Work out the finished part from the listing and answer in its coordinate system (mm). A direction names the side the tool comes from. Coordinates: 2 decimals unless noted, no trailing zeros. Loops run counter-clockwise (first coordinate to the right, second up) from the corner with the lowest first, then second, coordinate; pieces in that order, holes last. Notation, with made-up numbers: M 79.25,40 L 110.25,40 A14 ccw 110.25,51 Z; hole C 5.5,38 d9. An arc over 180 degrees is marked long. Write each question's results on one line, items separated by ' | '.
```python
from build123d import *

# Parameters (mm, degrees)
SZKIC1_W                                             = 119.8
SZKIC1_H                                             = 10
DODANIE_WYCI_GNI_CIE2_DEPTH                          = 30
SZKIC21_W                                            = 119.8
SZKIC21_H                                            = 10
DODANIE_WYCI_GNI_CIE3_DEPTH                          = 9.8
POG_BIENIE_WALCOWE_POD_M2_WKR_T_DO_CZ_CI_D           = 2.4
POG_BIENIE_WALCOWE_POD_M2_WKR_T_DO_CZ_CI_CBORE_D     = 5
POG_BIENIE_WALCOWE_POD_M2_WKR_T_DO_CZ_CI_CBORE_DEPTH = 1.6
SZKIC28_R                                            = 11.1
WYTNIJ_WYCI_GNI_CIE1_DEPTH                           = 7.2
WYTNIJ_WYCI_GNI_CIE4_DEPTH                           = 124.8
DODANIE_WYCI_GNI_CIE5_DEPTH                          = 119.8
SZKIC34_W                                            = 119.8
SZKIC34_H                                            = 10
DODANIE_WYCI_GNI_CIE6_DEPTH                          = 1.5


with BuildPart() as part:
    # Szkic1 → Dodanie-wyci_gni_cie2 (new body)
    with BuildSketch(Plane.XY):
        with Locations((1.59336777, 27.024849398)):
            Rectangle(SZKIC1_W, SZKIC1_H)
    extrude(amount=DODANIE_WYCI_GNI_CIE2_DEPTH)

    # Szkic21 → Dodanie-wyci_gni_cie3 (add)
    with BuildSketch(Plane(origin=(0, 32.024849398, 0), x_dir=(1, 0, 0), z_dir=(0, 1, 0))):
        with Locations((1.59336777, -5)):
            Rectangle(SZKIC21_W, SZKIC21_H)
    extrude(amount=DODANIE_WYCI_GNI_CIE3_DEPTH)

    # Pog_bienie walcowe pod M2 wkr_t do cz_ci (through all)
    with Locations(Plane(origin=(0, 22.024849398, 0), x_dir=(-1, 0, 0), z_dir=(0, -1, 0))):
        with Locations((-21.49336777, -4.88), (18.30663223, -4.88)):
            CounterBoreHole(POG_BIENIE_WALCOWE_POD_M2_WKR_T_DO_CZ_CI_D / 2, POG_BIENIE_WALCOWE_POD_M2_WKR_T_DO_CZ_CI_CBORE_D / 2, POG_BIENIE_WALCOWE_POD_M2_WKR_T_DO_CZ_CI_CBORE_DEPTH)

    # Szkic28 → Wytnij-wyci_gni_cie1 (cut)
    with BuildSketch(Plane.XZ.offset(-22.024849398)):
        with Locations(Location((38.49336777, 15, 0), (0, 0, 270))):
            Circle(SZKIC28_R)
    extrude(amount=-WYTNIJ_WYCI_GNI_CIE1_DEPTH, mode=Mode.SUBTRACT)

    # Szkic31 → Wytnij-wyci_gni_cie4 (cut)
    with BuildSketch(Plane(origin=(61.49336777, 0, 0), x_dir=(0, 0, -1), z_dir=(1, 0, 0))):
        Polygon((0, 41.824849398), (-0.096491228, 41.824849398), (0, 41.232541705), align=None)
    extrude(amount=-WYTNIJ_WYCI_GNI_CIE4_DEPTH, mode=Mode.SUBTRACT)

    # Szkic31_5 → Dodanie-wyci_gni_cie5 (add)
    with BuildSketch(Plane(origin=(61.49336777, 0, 0), x_dir=(0, 0, -1), z_dir=(1, 0, 0))):
        Polygon((0, 41.232541705), (0, 32.024849398), (1.5, 32.024849398), (0.275236278, 39.543014399), align=None)
    extrude(amount=-DODANIE_WYCI_GNI_CIE5_DEPTH)

    # Szkic34 → Dodanie-wyci_gni_cie6 (add)
    with BuildSketch(Plane(origin=(0, 0, 0), x_dir=(-1, 0, 0), z_dir=(0, 0, -1))):
        with Locations((-1.59336777, 27.024849398)):
            Rectangle(SZKIC34_W, SZKIC34_H)
    extrude(amount=DODANIE_WYCI_GNI_CIE6_DEPTH)


with BuildPart() as body_2:
    # Lustro2: mirrored copy
    add(part.part.mirror(Plane(origin=(-58.30663223, 22.024849398, 30), x_dir=(0, 0, 1), z_dir=(0, 1, 0))))


with BuildPart() as body_2_1:
    # Obiekt-Przenie_Kopiuj1: moved
    add(body_2.part.moved(Location((0, -41, 0))))


solid = body_2_1.part
```
1) Straight lines are drawn through the part: probe 1 along X at (y, z) = (-31.25, 4.88); probe 2 along Y at (x, z) = (-47, 24); probe 3 along Z at (x, y) = (36, -24). For each, find the intervals that lie inside material, in ascending order. Write a range as [from, to].
Check result:
probe 1: [-58.31, -19.51], [-17.11, 20.29], [22.69, 61.49] | probe 2: [-28.98, -18.98] | probe 3: [-1.5, 4.18], [25.82, 30]
2) Given pin 1 Ø11 at (x, z) = (38.5, 14.5) entering from +Y; pin 2 Ø10 at (x, z) = (-25.5, 23) entering from -Y; pin 3 Ø4 at (x, z) = (-18.31, 4.88) entering from +Y, each flat-ended and moving along its own axis, determine where each tip first touches the part or whether it passes through.
Check result:
pin 1: y = -26.18 | pin 2: y = -28.98 | pin 3: y = -20.58
3) Which of the six approach directions +Z, -Z, +X, -X, +Y, -Y give full straight-line access (tool end or side, diameter ignored) to faces 4 (the face through (1, -38.775, 5)), 5 (the face through (39, -26.175, 15)), 6 (the face through (1, -28.975, 20))?
Check result:
face 4: +Z, -Z, +X, -X, -Y | face 5: +Y | face 6: +Z, +X, -X, -Y
4) For a pull along X with two mould halves and no side action, classify faces 1 (the face through (61.493, -27, 11)), 2 (the face through (23.99, -19.76, 4.77)), 3 (the face through (2, -24, -1.5)) as released by +X, released by -X, zero draft, split by the parting line, or undercut.
Check result:
face 1: released by +X | face 2: undercut | face 3: zero draft
5) Find section B-B, the plane y = -24. Give the vertices of the cut face in (x, z).
Check result:
outline: M -58.31,-1.5 L 61.49,-1.5 L 61.49,30 L -58.31,30 Z; hole C -18.31,4.88 d2.4; hole C 21.49,4.88 d2.4; hole C 38.49,15 d22.2
6) Find section A-A, the plane z = 15. Give the vertices of the cut face in (x, y), and give its area (3 significant figures).
Check result:
outline: M -58.31,-28.98 L 61.49,-28.98 L 61.49,-18.98 L 49.59,-18.98 L 49.59,-26.18 L 27.39,-26.18 L 27.39,-18.98 L -58.31,-18.98 Z | area: 1,040 mm^2
7) Find section D-D, the plane y = -30.5. Give the vertices of the cut face in (x, z).
Check result:
outline: M -58.31,-1.25 L 61.49,-1.25 L 61.49,10 L -58.31,10 Z; hole C -18.31,4.88 d2.4; hole C 21.49,4.88 d2.4
8) Find section C-C, the plane x = 12. Give the vertices of the cut face in (y, z), and give its area (3 significant figures).
Check result:
outline: M -38.78,0.1 L -28.98,-1.5 L -18.98,-1.5 L -18.98,30 L -28.98,30 L -28.98,10 L -38.78,10 Z | area: 420 mm^2
